Design review of the part shown in the three views and the two pictorial views. Dimensions are in mm from the part's minimum x, y and z. A direction names the side the tool comes from. Round coordinates to 2 decimals unless told otherwise and drop trailing zeros. Order: outer loops, then holes, each group sorted by start corner. A loop starts at its lowest first (then second) coordinate and runs counter-clockwise, first axis right, second up. Notation, with made-up numbers: M -30,43.25 L 8,43.25 A15 cw 8,56.25 Z; hole C -7,61 d11. An arc over 180 degrees is marked long. Write each question's results on one line, items separated by ' | '. Start each with the question number.
Item 1: Take a section at B-B, the plane x = 9.5. Write out the cut boundary in (y, z).
Item 2: Take a section at A-A, the plane y = 6. Write out the cut boundary in (x, z) (1 decimal).
Item 3: Wall thickness on line 1 (Z direction, x = 16.5, y = 6.75); line 2 (Z direction, x = 10.75, y = 1.5); line 3 (X direction, y = 7, z = 1.5) (1 decimal): over which ranges is each line inside the solid? List them lowest first. Write a range as [from, to].
Item 4: Take a section at C-C, the plane y = 2. Write out the cut boundary in (x, z) (1 decimal).
Item 5: Clearance check with flat-ended pins moving along their axes: pin 1 (2 mm diameter, centred on y = 7, z = 8.5, fed in from +X); pin 2 (3 mm diameter, centred on y = 5, z = 8, fed in from +X); pin 3 (4 mm diameter, centred on x = 8, y = 5, fed in from -Z). State where each tip first meets the part, or that it passes through.
Item 6: Machinability: for the marked faces 1 and 2, which of the approach directions +Z, -Z, +X, -X, +Y, -Y give a long, thin tool a straight path to every point of the face, cutting with its end or side? Answer none if there is none.
Item 7: The part is to be moulded in two halves that separate along Y. For the marked faces 3, 4 and 5, say which applies: +Y half, -Y half, draft (parallel to the pull), parting line (faces both ways), or undercut.
Item 8: Take a section at D-D, the plane z = 1. Write out the cut boundary in (x, y).
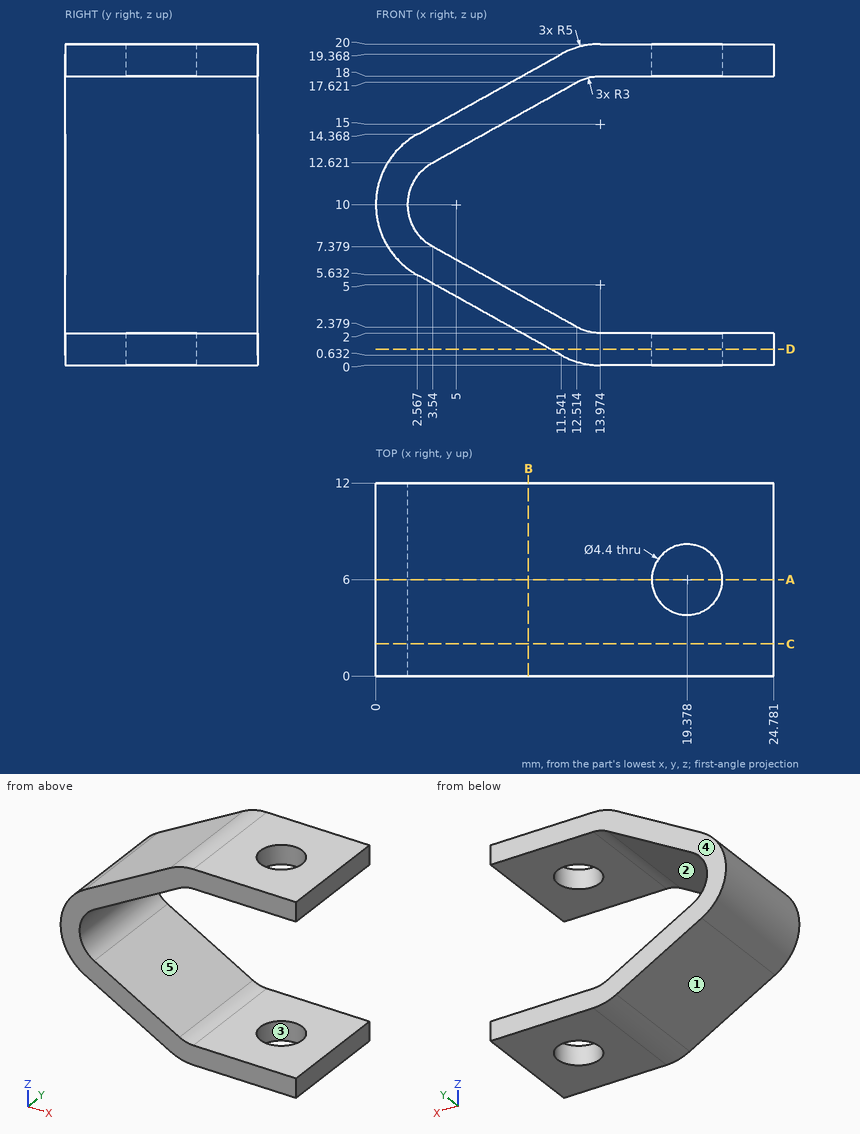
Results list:
1) outline: M 0,1.77 L 12,1.77 L 12,4.06 L 0,4.06 Z; M 0,15.94 L 12,15.94 L 12,18.23 L 0,18.23 Z
2) outline: M 2.6,5.6 L 11.5,0.6 A5 ccw 14,0 L 17.2,0 L 17.2,2 L 14,2 A3 cw 12.5,2.4 L 3.5,7.4 A3 cw 3.5,12.6 L 12.5,17.6 A3 cw 14,18 L 17.2,18 L 17.2,20 L 14,20 A5 ccw 11.5,19.4 L 2.6,14.4 A5 ccw Z; M 21.6,0 L 24.8,0 L 24.8,2 L 21.6,2 Z; M 21.6,18 L 24.8,18 L 24.8,20 L 21.6,20 Z
3) line 1: [0, 2], [18, 20] | line 2: [1.07, 3.36], [16.64, 18.93] | line 3: [10, 17.4], [21.3, 24.8]
4) outline: M 2.6,5.6 L 11.5,0.6 A5 ccw 14,0 L 24.8,0 L 24.8,2 L 14,2 A3 cw 12.5,2.4 L 3.5,7.4 A3 cw 3.5,12.6 L 12.5,17.6 A3 cw 14,18 L 24.8,18 L 24.8,20 L 14,20 A5 ccw 11.5,19.4 L 2.6,14.4 A5 ccw Z
5) pin 1: x = 3.34 | pin 2: x = 5.12 | pin 3: z = 1.49
6) face 1: -Z, -X, +Y, -Y | face 2: +X, +Y, -Y
7) face 3: undercut | face 4: +Y half | face 5: draft
8) outline: M 10.88,0 L 24.78,0 L 24.78,12 L 10.88,12 Z; hole C 19.38,6 d4.4
